from build123d import *

# Parameters (mm, degrees)
F0_R     = 60
F1_DEPTH = 30


with BuildPart() as f1:
    # F0 (on Top) → F1 (new body)
    with BuildSketch(Plane.XY):
        with BuildLine():
            Line((-130, -80), (-60, -80))
            ThreePointArc((-60, -80), (0, -100), (60, -80))
            Line((60, -80), (130, -80))
            Line((130, -80), (130, -30))
            ThreePointArc((130, -30), (150, 0), (130, 30))
            Line((130, 30), (130, 80))
            Line((130, 80), (60, 80))
            ThreePointArc((60, 80), (0, 100), (-60, 80))
            Line((-60, 80), (-130, 80))
            Line((-130, 80), (-130, 30))
            ThreePointArc((-130, 30), (-150, 0), (-130, -30))
            Line((-130, -30), (-130, -80))
        make_face()
        with BuildLine():
            Line((-115, -55), (-115, 55))
            ThreePointArc((-115, 55), (-112.071068, 62.071068), (-105, 65))
            Line((-105, 65), (-95, 65))
            ThreePointArc((-95, 65), (-87.928932, 62.071068), (-85, 55))
            Line((-85, 55), (-85, -55))
            ThreePointArc((-85, -55), (-87.928932, -62.071068), (-95, -65))
            Line((-95, -65), (-105, -65))
            ThreePointArc((-105, -65), (-112.071068, -62.071068), (-115, -55))
        make_face(mode=Mode.SUBTRACT)
        Circle(F0_R, mode=Mode.SUBTRACT)
        with BuildLine():
            ThreePointArc((85, 55), (87.928932, 62.071068), (95, 65))
            Line((95, 65), (105, 65))
            ThreePointArc((105, 65), (112.071068, 62.071068), (115, 55))
            Line((115, 55), (115, -55))
            ThreePointArc((115, -55), (112.071068, -62.071068), (105, -65))
            Line((105, -65), (95, -65))
            ThreePointArc((95, -65), (87.928932, -62.071068), (85, -55))
            Line((85, -55), (85, 55))
        make_face(mode=Mode.SUBTRACT)
    extrude(amount=F1_DEPTH)


solid = f1.part
For this review, take the finished solid that the model builds, in its own axes (mm). A direction names the side the tool comes from. Give positions to 0.01 mm unless a question says otherwise; leave off trailing zeros. Loops run counter-clockwise (first coordinate to the right, second up) from the corner with the lowest first, then second, coordinate; pieces in that order, holes last. Notation, with made-up numbers: M 28.25,-9 L 36.25,-9 A22 cw 36.25,3 Z; hole C 14,53.25 d5. An arc over 180 degrees is marked long. Put each result on its own line as item: value. Start each with the question number.
(1) Machinability: for faces 4 (the flat face through (-130, -55, 15)), 5 (the flat face through (-95, 80, 15)), 6 (the cylindrical face through (-112.15, 61.99, 14.79)), which of the approach directions +Z, -Z, +X, -X, +Y, -Y give a long, thin tool a straight path to every point of the face, cutting with its end or side? Answer none if there is none.
(2) Wall thickness on L1, parallel to Y at x = 0, z = 8.75; L2, parallel to Y at x = 103, z = 7; L3, parallel to X at y = -49.5, z = 23.5: over which ranges is each line inside the solid? List them lowest first.
(3) Add section D-D, the plane x = 0. Write out the cut boundary in (y, z).
(4) Add section B-B, the plane y = 0. Write out the cut boundary in (x, z).
(5) The part is to be moulded in two halves that separate along Y. For faces 1 (the flat face through (-2, 68, 0)), 2 (the flat face through (-95, -80, 15)), 3 (the cylindrical face through (112.15, -61.99, 14.79)), say which applies: +Y half, -Y half, draft (parallel to the pull), parting line (faces both ways), or undercut.
(6) Add section C-C, the plane z = 20. Give the number of separate pieces and of enclosed holes in the cut face, then the cut area to 3 significant figures.
(7) Add section A-A, the plane x = -98.5. Write out the cut boundary in (y, z), then the cut area to 3 significant figures.
(8) For pin 1 (9 mm diameter, centred on y = -56.5, z = 18, fed in from +X); pin 2 (3 mm diameter, centred on x = -101.5, z = 22, fed in from +Y); pin 3 (5 mm diameter, centred on y = -19, z = 7, fed in from +X), all flat-tipped, find the tip position at first contact; note any pin that passes through.
Result:
1. face 4: +Z, -Z, -X, -Y
1. face 5: +Z, -Z, -X, +Y
1. face 6: +Z, -Z
2. L1: y = -100 to -60, 60 to 100
2. L2: y = -80 to -65, 65 to 80
2. L3: x = -130 to -115, -85 to -33.91, 33.91 to 85, 115 to 130
3. outline: M -100,0 L -60,0 L -60,30 L -100,30 Z; M 60,0 L 100,0 L 100,30 L 60,30 Z
4. outline: M -150,0 L -115,0 L -115,30 L -150,30 Z; M -85,0 L -60,0 L -60,30 L -85,30 Z; M 60,0 L 85,0 L 85,30 L 60,30 Z; M 115,0 L 150,0 L 150,30 L 115,30 Z
5. face 1: draft
5. face 2: -Y half
5. face 3: undercut
6. separate pieces: 1
6. enclosed holes: 3
6. area: 27,700 mm^2
7. outline: M -80,0 L -65,0 L -65,30 L -80,30 Z; M 65,0 L 80,0 L 80,30 L 65,30 Z
7. area: 900 mm^2
8. pin 1: stops at x = 130
8. pin 2: stops at y = 80
8. pin 3: stops at x = 145.5
